Part model, mm, in its own coordinate system. A direction names the side the tool comes from. Give positions to 0.01 mm unless a question says otherwise; leave off trailing zeros. Write each loop counter-clockwise with the first axis right and the second up, starting at its lowest first coordinate (ties: lowest second). Pieces come first, ordered by that corner, then holes.
```python
from build123d import *

# Parameters (mm, degrees)
SKETCH1_W           = 10
SKETCH1_H           = 60
BOSS_EXTRUDE1_DEPTH = 7
SKETCH2_W           = 10
SKETCH2_H           = 13
CUT_EXTRUDE1_DEPTH  = 4
SKETCH3_R           = 2
CUT_EXTRUDE2_DEPTH  = 4
SKETCH4_R           = 1.5
CUT_EXTRUDE3_DEPTH  = 14
BOSS_EXTRUDE2_DEPTH = 2


with BuildPart() as part:
    # Sketch1 → Boss-Extrude1 (new body)
    with BuildSketch(Plane(origin=(0, 0, 0), x_dir=(1, 0, 0), z_dir=(0, 1, 0))):
        Rectangle(SKETCH1_W, SKETCH1_H)
    extrude(amount=BOSS_EXTRUDE1_DEPTH)

    # Sketch2 → Cut-Extrude1 (cut)
    with BuildSketch(Plane(origin=(0, 7, 0), x_dir=(1, 0, 0), z_dir=(0, 1, 0))):
        with Locations((0, 23.5)):
            Rectangle(SKETCH2_W, SKETCH2_H)
    extrude(amount=-CUT_EXTRUDE1_DEPTH, mode=Mode.SUBTRACT)

    # Sketch3 → Cut-Extrude2 (cut)
    with BuildSketch(Plane(origin=(0, 3, 0), x_dir=(1, 0, 0), z_dir=(0, 1, 0))):
        with Locations((0, 26)):
            Circle(SKETCH3_R)
    extrude(amount=-CUT_EXTRUDE2_DEPTH, mode=Mode.SUBTRACT)

    # Sketch4 → Cut-Extrude3 (cut)
    with BuildSketch(Plane(origin=(0, 0, 0), x_dir=(1, 0, 0), z_dir=(0, 1, 0))):
        Circle(SKETCH4_R)
        with Locations((0, -20)):
            Circle(SKETCH4_R)
    extrude(amount=CUT_EXTRUDE3_DEPTH, mode=Mode.SUBTRACT)

    # Sketch5 → Boss-Extrude2 (add)
    with BuildSketch(Plane(origin=(5, 0, 0), x_dir=(0, 0, -1), z_dir=(1, 0, 0))):
        Polygon((-30, 7), (-30, 0), (30, 0), (30, 3), (17, 3), (17, 7), align=None)
    extrude(amount=BOSS_EXTRUDE2_DEPTH)


solid = part.part
```
1) Saw through at C-C, the plane x = 0. Write the cut outline in (y, z).
Answers follow:
outline: (0, -30) - (3, -30) - (3, -28) - (0, -28) - close; (0, -24) - (3, -24) - (3, -17) - (7, -17) - (7, -1.5) - (0, -1.5) - close; (0, 1.5) - (7, 1.5) - (7, 18.5) - (0, 18.5) - close; (0, 21.5) - (7, 21.5) - (7, 30) - (0, 30) - close
2) Two-plate mould, pull along X, no slides. Class faces 1 (the face through (-1.5, 3.45, -0.07)), 2 (the face through (7, 4, 0)), 3 (the face through (1, 3, -24)): +X half, -X half, draft (parallel to the pull), parting line (faces both ways), or undercut.
Answers follow:
face 1: undercut
face 2: +X half
face 3: draft
3) Wall check: L1, parallel to X at y = 5.75, z = 20; L2, parallel to X at y = 1.7, z = -26; L3, parallel to Z at x = -3.75, y = 6.75. Give the ranges that are in metal, low to high.
Answers follow:
L1: x = -5 to -1.5, 1.5 to 7
L2: x = -5 to -2, 2 to 7
L3: z = -17 to 30
4) Pin check, flat tips, straight feed: pin 1 Ø3 at (x, z) = (0, -26) entering from -Y; pin 2 Ø2 at (x, y) = (3, 5) entering from -Z. Stop position of each tip, or through.
Answers follow:
pin 1: passes through
pin 2: stops at z = -17
5) 3-axis set-ups, long thin cutter, end or side, ignore diameter. For faces 4 (the face through (-0.195, 3.451, 18.513)), 5 (the face through (1, 5, -17)): which of +Z, -Z, +X, -X, +Y, -Y reach the whole face in a straight line?
Answers follow:
face 4: +Y, -Y
face 5: -Z, +X, -X, +Y
6) Saw through at A-A, the plane z = -26. Write the cut outline in (x, y).
Answers follow:
outline: (-5, 0) - (-2, 0) - (-2, 3) - (-5, 3) - close; (2, 0) - (7, 0) - (7, 3) - (2, 3) - close
7) Saw through at D-D, the plane y = 4.5. Write the cut outline in (x, z), then the cut area to 3 significant figures.
Answers follow:
outline: (-5, -17) - (7, -17) - (7, 30) - (-5, 30) - close; hole circle Ø3 at (0, 0); hole circle Ø3 at (0, 20)
area: 550 mm2
8) Saw through at B-B, the plane y = 1. Write the cut outline in (x, z), then the cut area to 3 significant figures.
Answers follow:
outline: (-5, -30) - (7, -30) - (7, 30) - (-5, 30) - close; hole circle Ø4 at (0, -26); hole circle Ø3 at (0, 0); hole circle Ø3 at (0, 20)
area: 693 mm2
